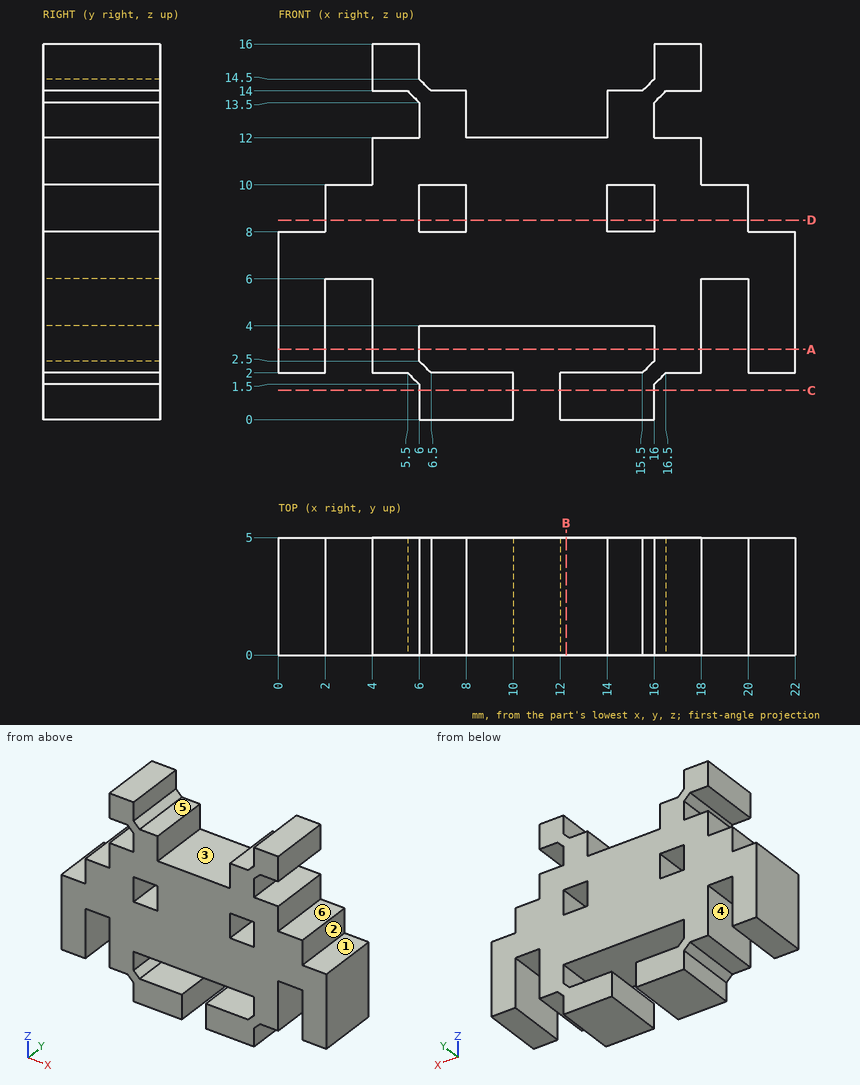
Job drawing, mm, ordinate dimensions from the low corner. One solid piece. A direction names the side the tool comes from. Give positions to 0.01 mm unless a question says otherwise; leave off trailing zeros. Loops run counter-clockwise (first coordinate to the right, second up) from the corner with the lowest first, then second, coordinate; pieces in that order, holes last. Notation, with made-up numbers: (-4.5, 34.25) -> (7.5, 34.25) arc R20 ccw to (7.5, 51.25) -> close; hole circle Ø7 at (11, 40). An arc over 180 degrees is marked (long way). Write each question's results on one line, items separated by ' | '. Start each with the question number.
Q1. Band-saw the part on A-A on z = 3. List the corners of the cut face in (x, y).
Q2. Band-saw the part on C-C on z = 1.25. List the corners of the cut face in (x, y).
Q3. Pull direction X, two halves, no side cores. Call the marked faces 1, 2 and 3: +X half, -X half, draft (parallel to the pull), parting line (faces both ways), or undercut.
Q4. Band-saw the part on D-D on z = 8.5. List the corners of the cut face in (x, y).
Q5. Wall check: L1, parallel to X at y = 3.85, z = 2.75; L2, parallel to Z at x = 6.75, y = 0.8; L3, parallel to Z at x = 17, y = 2.3. Give the ranges that are in metal, low to high.
Q6. Which spindle directions (+Z, -Z, +X, -X, +Y, -Y) get a long thin tool onto all of the face, cutting with end or side? Do the marked faces 4, 5 and 6. Say none if no direction does.
Q7. Band-saw the part on B-B on x = 12.25. List the corners of the cut face in (y, z), plus the area to 3 significant figures.
Q8. Pin check, flat tips, straight feed: P1, Ø1.2, axis at x = 7.5, y = 1.5, coming from the +Z side; P2, Ø1.6, axis at y = 3, z = 13, coming from the +X side; P3, Ø2, axis at y = 1.5, z = 12, coming from the +X side. Stop position of each tip, or through.
Results are:
1) outline: (0, 0) -> (2, 0) -> (2, 5) -> (0, 5) -> close; (4, 0) -> (6, 0) -> (6, 5) -> (4, 5) -> close; (16, 0) -> (18, 0) -> (18, 5) -> (16, 5) -> close; (20, 0) -> (22, 0) -> (22, 5) -> (20, 5) -> close
2) outline: (6, 0) -> (10, 0) -> (10, 5) -> (6, 5) -> close; (12, 0) -> (16, 0) -> (16, 5) -> (12, 5) -> close
3) face 1: draft | face 2: +X half | face 3: undercut
4) outline: (2, 0) -> (6, 0) -> (6, 5) -> (2, 5) -> close; (8, 0) -> (14, 0) -> (14, 5) -> (8, 5) -> close; (16, 0) -> (20, 0) -> (20, 5) -> (16, 5) -> close
5) L1: x = 0 to 2, 4 to 6, 16 to 18, 20 to 22 | L2: z = 0 to 2, 4 to 8, 10 to 14 | L3: z = 2 to 12, 14 to 16
6) face 4: -Z, +Y, -Y | face 5: +Z, +Y, -Y | face 6: +Z, +X, +Y, -Y
7) outline: (0, 0) -> (5, 0) -> (5, 2) -> (0, 2) -> close; (0, 4) -> (5, 4) -> (5, 12) -> (0, 12) -> close | area: 50.0 mm²
8) P1: stops at z = 14 | P2: stops at x = 16.3 | P3: stops at x = 18
